Here's how the part is built. I have some questions about the finished solid (model axes, mm). Give positions to 0.01 mm unless a question says otherwise; leave off trailing zeros. Write each loop counter-clockwise with the first axis right and the second up, starting at its lowest first coordinate (ties: lowest second). Pieces come first, ordered by that corner, then holes. Notation, with made-up numbers: (74.5, 18) -> (117.5, 18) arc R14 cw to (117.5, 42) -> close; hole circle Ø11 at (-6, 77.25). An arc over 180 degrees is marked (long way). Return JSON: item names as keys, results as strings.
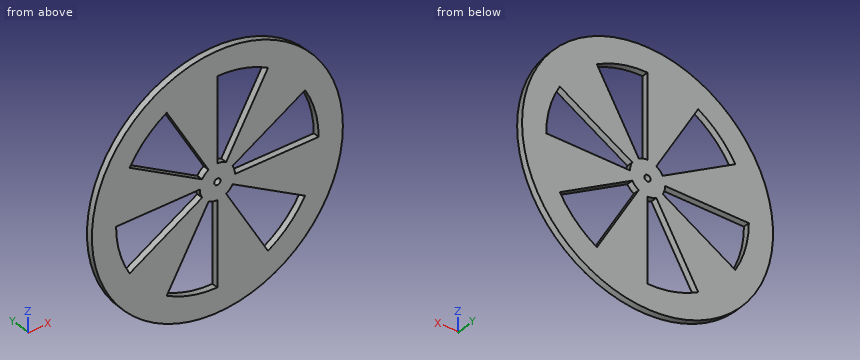
from build123d import *

# Parameters (mm, degrees)
F0_R     = 63.5
F0_R_2   = 1.5875
F1_DEPTH = 3.175
F2_R     = 1.5875
F3_DEPTH = 3.175


with BuildPart() as f1:
    # F0 (on Front) → F1 (new body)
    with BuildSketch(Plane.XZ):
        Circle(F0_R)
        with BuildLine():
            ThreePointArc((44.386194, 25.626381), (49.506367, 13.265191), (51.252762, 0))
            ThreePointArc((51.252762, 0), (49.506367, -13.265191), (44.386194, -25.626381))
            ThreePointArc((44.386194, -25.626381), (36.241176, -36.241176), (25.626381, -44.386194))
            ThreePointArc((25.626381, -44.386194), (13.265191, -49.506367), (0, -51.252762))
            ThreePointArc((0, -51.252762), (-13.265191, -49.506367), (-25.626381, -44.386194))
            ThreePointArc((-25.626381, -44.386194), (-36.241176, -36.241176), (-44.386194, -25.626381))
            ThreePointArc((-44.386194, -25.626381), (-49.506367, -13.265191), (-51.252762, 0))
            ThreePointArc((-51.252762, 0), (-49.506367, 13.265191), (-44.386194, 25.626381))
            ThreePointArc((-44.386194, 25.626381), (-36.241176, 36.241176), (-25.626381, 44.386194))
            ThreePointArc((-25.626381, 44.386194), (-13.265191, 49.506367), (0, 51.252762))
            ThreePointArc((0, 51.252762), (13.265191, 49.506367), (25.626381, 44.386194))
            ThreePointArc((25.626381, 44.386194), (36.241176, 36.241176), (44.386194, 25.626381))
        make_face(mode=Mode.SUBTRACT)
        with BuildLine():
            Line((-7.698966, 4.445), (-44.386194, 25.626381))
            ThreePointArc((-44.386194, 25.626381), (-49.506367, 13.265191), (-51.252762, 0))
            Line((-51.252762, 0), (-8.89, 0))
            ThreePointArc((-8.89, 0), (-8.587081, 2.300901), (-7.698966, 4.445))
        make_face()
        with BuildLine():
            Line((0, 8.89), (0, 51.252762))
            ThreePointArc((0, 51.252762), (-13.265191, 49.506367), (-25.626381, 44.386194))
            Line((-25.626381, 44.386194), (-4.445, 7.698966))
            ThreePointArc((-4.445, 7.698966), (-2.300901, 8.587081), (0, 8.89))
        make_face()
        with BuildLine():
            Line((7.698966, 4.445), (44.386194, 25.626381))
            ThreePointArc((44.386194, 25.626381), (36.241176, 36.241176), (25.626381, 44.386194))
            Line((25.626381, 44.386194), (4.445, 7.698966))
            ThreePointArc((4.445, 7.698966), (6.286179, 6.286179), (7.698966, 4.445))
        make_face()
        with BuildLine():
            ThreePointArc((44.386194, -25.626381), (49.506367, -13.265191), (51.252762, 0))
            Line((51.252762, 0), (8.89, 0))
            ThreePointArc((8.89, 0), (8.587081, -2.300901), (7.698966, -4.445))
            Line((7.698966, -4.445), (44.386194, -25.626381))
        make_face()
        with BuildLine():
            ThreePointArc((0, -51.252762), (13.265191, -49.506367), (25.626381, -44.386194))
            Line((25.626381, -44.386194), (4.445, -7.698966))
            ThreePointArc((4.445, -7.698966), (2.300901, -8.587081), (0, -8.89))
            Line((0, -8.89), (0, -51.252762))
        make_face()
        with BuildLine():
            ThreePointArc((-44.386194, -25.626381), (-36.241176, -36.241176), (-25.626381, -44.386194))
            Line((-25.626381, -44.386194), (-4.445, -7.698966))
            ThreePointArc((-4.445, -7.698966), (-6.286179, -6.286179), (-7.698966, -4.445))
            Line((-7.698966, -4.445), (-44.386194, -25.626381))
        make_face()
        with BuildLine():
            ThreePointArc((7.698966, -4.445), (8.587081, -2.300901), (8.89, 0))
            ThreePointArc((8.89, 0), (8.587081, 2.300901), (7.698966, 4.445))
            ThreePointArc((7.698966, 4.445), (6.286179, 6.286179), (4.445, 7.698966))
            ThreePointArc((4.445, 7.698966), (2.300901, 8.587081), (0, 8.89))
            ThreePointArc((0, 8.89), (-2.300901, 8.587081), (-4.445, 7.698966))
            ThreePointArc((-4.445, 7.698966), (-6.286179, 6.286179), (-7.698966, 4.445))
            ThreePointArc((-7.698966, 4.445), (-8.587081, 2.300901), (-8.89, 0))
            ThreePointArc((-8.89, 0), (-8.587081, -2.300901), (-7.698966, -4.445))
            ThreePointArc((-7.698966, -4.445), (-6.286179, -6.286179), (-4.445, -7.698966))
            ThreePointArc((-4.445, -7.698966), (-2.300901, -8.587081), (0, -8.89))
            ThreePointArc((0, -8.89), (2.300901, -8.587081), (4.445, -7.698966))
            ThreePointArc((4.445, -7.698966), (6.286179, -6.286179), (7.698966, -4.445))
        make_face()
        Circle(F0_R_2, mode=Mode.SUBTRACT)
    extrude(amount=F1_DEPTH)

    # F2 (on face) → F3 (cut)
    with BuildSketch(Plane.XZ.offset(3.175)):
        Circle(F2_R)
    extrude(amount=-F3_DEPTH, mode=Mode.SUBTRACT)


solid = f1.part
1. Suppose I cut it at D-D, the plane z = -15.5. List the corners of the cut face in (x, y) for me (3 decimals).
Taken from the geometry:
{"outline": "(-61.579, -3.175) -> (-48.853, -3.175) -> (-48.853, 0) -> (-61.579, 0) -> close; (-26.847, -3.175) -> (-8.949, -3.175) -> (-8.949, 0) -> (-26.847, 0) -> close; (0, -3.175) -> (8.949, -3.175) -> (8.949, 0) -> (0, 0) -> close; (26.847, -3.175) -> (61.579, -3.175) -> (61.579, 0) -> (26.847, 0) -> close"}
2. For pin 1 Ø1 at (x, y) = (40.5, -1) entering from +Z; pin 2 Ø1 at (y, z) = (-2, -48) entering from -X; pin 3 Ø1.6 at (x, y) = (-19.5, -2) entering from -Z, each with a flat end and sliding along its axis, tell me the tip position at first contact or that it passes through.
Taken from the geometry:
{"pin 1": "stops at z = 49.32", "pin 2": "stops at x = -42.14", "pin 3": "stops at z = -60.68"}
3. Suppose I cut it at C-C, the plane x = -13. List the corners of the cut face in (y, z) for me (3 decimals), and give its area (3 significant figures).
Taken from the geometry:
{"outline": "(-3.175, -62.155) -> (0, -62.155) -> (0, -49.577) -> (-3.175, -49.577) -> close; (-3.175, -22.517) -> (0, -22.517) -> (0, -7.506) -> (-3.175, -7.506) -> close; (-3.175, 0) -> (0, 0) -> (0, 7.506) -> (-3.175, 7.506) -> close; (-3.175, 22.517) -> (0, 22.517) -> (0, 62.155) -> (-3.175, 62.155) -> close", "area": "237 mm²"}
4. Suppose I cut it at B-B, the plane z = 39. List the corners of the cut face in (x, y) for me (3 decimals), and give its area (3 significant figures).
Taken from the geometry:
{"outline": "(-50.112, -3.175) -> (-33.254, -3.175) -> (-33.254, 0) -> (-50.112, 0) -> close; (-22.517, -3.175) -> (0, -3.175) -> (0, 0) -> (-22.517, 0) -> close; (22.517, -3.175) -> (50.112, -3.175) -> (50.112, 0) -> (22.517, 0) -> close", "area": "213 mm²"}
5. Suppose I cut it at A-A, the plane y = -1.6. List the corners of the cut face in (x, z) for me (1 decimal).
Taken from the geometry:
{"outline": "circle Ø127 at (0, 0); hole (-51.3, 0) arc R51.3 ccw to (-44.4, -25.6) -> (-7.7, -4.4) arc R8.9 cw to (-8.9, 0) -> close; hole (-44.4, 25.6) -> (-7.7, 4.4) arc R8.9 cw to (-4.4, 7.7) -> (-25.6, 44.4) arc R51.3 ccw to start; hole (-25.6, -44.4) arc R51.3 ccw to (0, -51.3) -> (0, -8.9) arc R8.9 cw to (-4.4, -7.7) -> close; hole circle Ø3.2 at (0, 0); hole (0, 8.9) arc R8.9 cw to (4.4, 7.7) -> (25.6, 44.4) arc R51.3 ccw to (0, 51.3) -> close; hole (4.4, -7.7) -> (25.6, -44.4) arc R51.3 ccw to (44.4, -25.6) -> (7.7, -4.4) arc R8.9 cw to start; hole (7.7, 4.4) arc R8.9 cw to (8.9, 0) -> (51.3, 0) arc R51.3 ccw to (44.4, 25.6) -> close"}
6. If I drill on line 1 (X direction, y = -1.05, z = -8); line 2 (X direction, y = -2, z = 12.5); line 3 (X direction, y = -1.95, z = 43), over which ranges is the centre line in solid material (lowest first)? Write a range as [from, to].
Taken from the geometry:
{"line 1": "x = [-62.99, -50.62], [-13.86, -4.62], [-3.88, 4.62], [13.86, 62.99]", "line 2": "x = [-62.26, -21.65], [-7.22, 0], [7.22, 21.65], [49.71, 62.26]", "line 3": "x = [-46.73, -27.89], [-24.83, 0], [24.83, 46.73]"}
